Build history of the part. All positions in model axes, mm. Round coordinates to 2 decimals unless told otherwise and drop trailing zeros. Write each loop counter-clockwise with the first axis right and the second up, starting at its lowest first coordinate (ties: lowest second). Pieces come first, ordered by that corner, then holes. Notation, with made-up numbers: M 82,17.25 L 131,17.25 A21 cw 131,24.25 Z; hole C 49,21 d10. An arc over 180 degrees is marked long. One line per item, written item: value. Start each with the question number.
```python
from build123d import *

# Parameters (mm, degrees)
F0_W      = 177.8
F0_H      = 76.2
F1_DEPTH  = 31.75
F2_W      = 19.05
F2_H      = 76.2
F3_DEPTH  = 63.5
F4_W      = 107.95
F4_H      = 38.1
F5_DEPTH  = 31.751
F6_W      = 107.95
F6_H      = 19.05
F7_DEPTH  = 12.7
F8_W      = 76.2
F8_H      = 31.75
F9_DEPTH  = 50.8
F11_D     = 6.5278
F11_DEPTH = 12.7
F11_TIP   = 1.9611489744
F14_D     = 7.9375
F15_W     = 19.05
F15_H     = 19.05
F15_R     = 3.2639
F12_W     = 19.05
F12_H     = 19.05
F12_R     = 3.2639
F16_DEPTH = 107.95
F18_D     = 4.9784
F19_W     = 76.2
F19_H     = 95.25
F19_R     = 2.4892
F19_R_2   = 3.96875
F20_DEPTH = 1.27
F22_D     = 6.9088
F22_DEPTH = 24.3416666667
F22_TIP   = 2.0756129224


with BuildPart() as f1:
    # F0 (on Top) → F1 (new body)
    with BuildSketch(Plane.XY):
        with Locations((88.9, 38.1)):
            Rectangle(F0_W, F0_H)
    extrude(amount=F1_DEPTH)

    # F2 (on face) → F3 (join)
    with BuildSketch(Plane.XY.offset(31.75)):
        with Locations((9.525, 38.1)):
            Rectangle(F2_W, F2_H)
    extrude(amount=F3_DEPTH)

    # F4 (on face) → F5 (cut, through all)
    with BuildSketch(Plane.XY.offset(31.75)):
        with Locations((73.025, 38.1)):
            Rectangle(F4_W, F4_H)
    extrude(amount=-F5_DEPTH, mode=Mode.SUBTRACT)

    # F6 (on face) → F7 (cut)
    with BuildSketch(Plane(origin=(0, 0, 0), x_dir=(1, 0, 0), z_dir=(0, 0, -1))):
        with Locations((73.025, -9.525)):
            Rectangle(F6_W, F6_H)
        with Locations((73.025, -66.675)):
            Rectangle(F6_W, F6_H)
    extrude(amount=-F7_DEPTH, mode=Mode.SUBTRACT)

    # F8 (on face) → F9 (cut)
    with BuildSketch(Plane.YZ.offset(177.8)):
        with Locations((38.1, 15.875)):
            Rectangle(F8_W, F8_H)
    extrude(amount=-F9_DEPTH, mode=Mode.SUBTRACT)

    # F11
    with Locations(Plane.YZ.offset(127)):
        with Locations((66.675, 22.225), (9.525, 22.225)):
            Hole(F11_D / 2, depth=F11_DEPTH)
            with Locations((0, 0, -(F11_DEPTH + F11_TIP / 2))):  # 118° drill point
                Cone(0, F11_D / 2, F11_TIP, mode=Mode.SUBTRACT)

    # F14 (through all)
    with Locations(Plane(origin=(0, 0, 0), x_dir=(0, -1, 0), z_dir=(-1, 0, 0))):
        with Locations((-38.1, 63.5)):
            Hole(F14_D / 2)

    # F15 (on face) + F12 (on face) → F16 (cut)
    with BuildSketch(Plane.YZ.offset(127)):
        with Locations((66.675, 22.225)):
            Rectangle(F15_W, F15_H)
        with Locations((66.675, 22.225)):
            Circle(F15_R, mode=Mode.SUBTRACT)
        with Locations((9.525, 22.225)):
            Rectangle(F15_W, F15_H)
        with Locations((9.525, 22.225)):
            Circle(F15_R, mode=Mode.SUBTRACT)
        with Locations((9.525, 22.225)):
            Circle(F15_R)
    with BuildSketch(Plane.YZ.offset(127)):
        with Locations((66.675, 22.225)):
            Rectangle(F12_W, F12_H)
        with Locations((66.675, 22.225)):
            Circle(F12_R, mode=Mode.SUBTRACT)
        with Locations((66.675, 22.225)):
            Circle(F12_R)
    extrude(amount=-F16_DEPTH, mode=Mode.SUBTRACT)

    # F18 (through all)
    with Locations(Plane.YZ.offset(19.05)):
        with Locations((6.35, 25.4), (12.7, 19.05), (63.5, 19.05), (69.85, 25.4)):
            Hole(F18_D / 2)

    # F19 (on face) → F20 (cut)
    with BuildSketch(Plane(origin=(0, 0, 0), x_dir=(0, -1, 0), z_dir=(-1, 0, 0))):
        with Locations((-38.1, 47.625)):
            Rectangle(F19_W, F19_H)
        with Locations((-63.5, 19.05)):
            Circle(F19_R, mode=Mode.SUBTRACT)
        with Locations((-69.85, 25.4)):
            Circle(F19_R, mode=Mode.SUBTRACT)
        with Locations((-12.7, 19.05)):
            Circle(F19_R, mode=Mode.SUBTRACT)
        with Locations((-6.35, 25.4)):
            Circle(F19_R, mode=Mode.SUBTRACT)
        with Locations((-38.1, 63.5)):
            Circle(F19_R_2, mode=Mode.SUBTRACT)
    extrude(amount=-F20_DEPTH, mode=Mode.SUBTRACT)

    # F22
    with Locations(Plane(origin=(0, 0, 0), x_dir=(1, 0, 0), z_dir=(0, 0, -1))):
        with Locations((10.16, -38.1)):
            Hole(F22_D / 2, depth=F22_DEPTH)
            with Locations((0, 0, -(F22_DEPTH + F22_TIP / 2))):  # 118° drill point
                Cone(0, F22_D / 2, F22_TIP, mode=Mode.SUBTRACT)


solid = f1.part
```
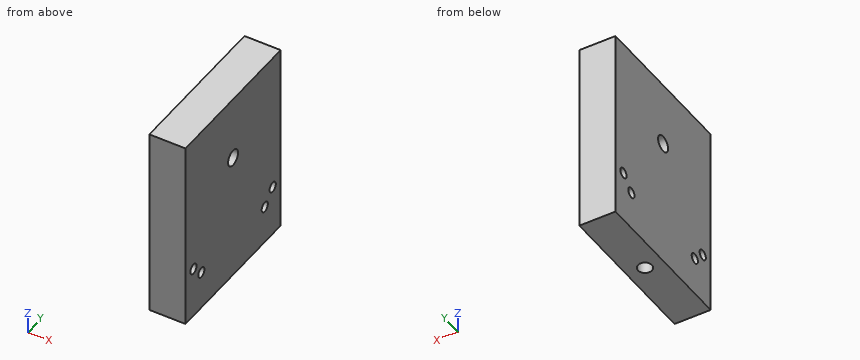
Item 1: Cut at A-A, the plane z = 18. Write the cut outline in (x, y), plus the area to 3 significant figures.
Item 2: Cut at B-B, the plane y = 69.85. Write the cut outline in (x, z), plus the area to 3 significant figures.
Item 3: Cut at D-D, the plane x = 16.75. Write the cut outline in (y, z), plus the area to 3 significant figures.
Item 4: Drill centre lines: line 1 (Z direction, x = 9, y = 6.35); line 2 (Y direction, x = 10.16, z = 15); line 3 (Y direction, x = 16, z = 23.5). Where is each one in solid material? Low to high.
Item 5: Drop flat-ended pins along their axis: pin 1 (4 mm diameter, centred on y = 69.85, z = 25.4, fed in from +X); pin 2 (5.5 mm diameter, centred on y = 12.7, z = 19.05, fed in from +X). Give the stop position or say it passes through.
Item 6: Cut at C-C, the plane z = 63.5. Write the cut outline in (x, y), plus the area to 3 significant figures.
Computed values:
1. outline: M 1.27,0 L 19.05,0 L 19.05,10.44 L 1.27,10.44 Z; M 1.27,14.96 L 19.05,14.96 L 19.05,61.24 L 1.27,61.24 Z; M 1.27,65.76 L 19.05,65.76 L 19.05,76.2 L 1.27,76.2 Z; hole C 10.16,38.1 d6.91
1. area: 1,160 mm2
2. outline: M 1.27,0 L 19.05,0 L 19.05,22.91 L 1.27,22.91 Z; M 1.27,27.89 L 19.05,27.89 L 19.05,95.25 L 1.27,95.25 Z
2. area: 1,610 mm2
3. outline: M 0,0 L 76.2,0 L 76.2,95.25 L 0,95.25 Z; hole C 6.35,25.4 d4.98; hole C 12.7,19.05 d4.98; hole C 38.1,63.5 d7.94; hole C 63.5,19.05 d4.98; hole C 69.85,25.4 d4.98
3. area: 7,130 mm2
4. line 1: z = 0 to 22.91, 27.89 to 95.25
4. line 2: y = 0 to 34.65, 41.55 to 76.2
4. line 3: y = 0 to 4.74, 7.96 to 68.24, 71.46 to 76.2
5. pin 1: passes through
5. pin 2: stops at x = 19.05
6. outline: M 1.27,0 L 19.05,0 L 19.05,34.13 L 1.27,34.13 Z; M 1.27,42.07 L 19.05,42.07 L 19.05,76.2 L 1.27,76.2 Z
6. area: 1,210 mm2
